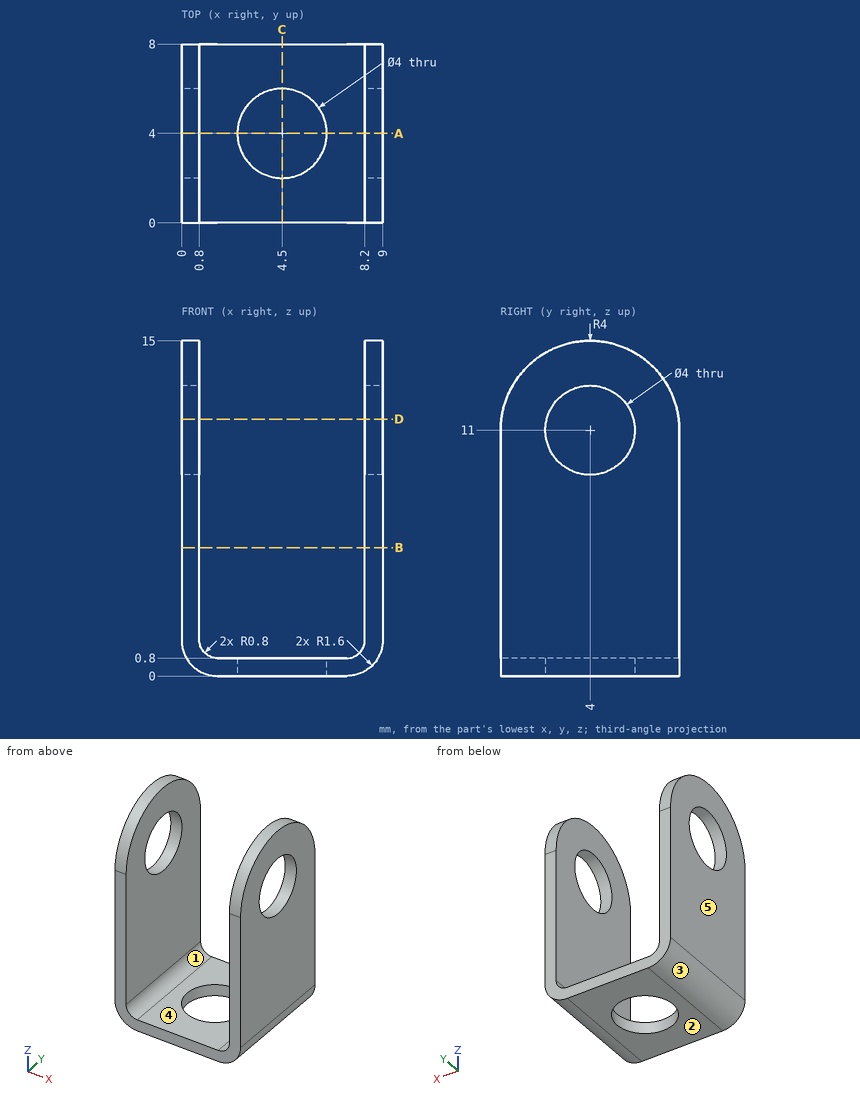
Could you check a few things on this drawing? It's one solid part, dimensions in mm from its lowest x, y, z. A direction names the side the tool comes from. Give positions to 0.01 mm unless a question says otherwise; leave off trailing zeros. Order: outer loops, then holes, each group sorted by start corner. A loop starts at its lowest first (then second) coordinate and runs counter-clockwise, first axis right, second up. Notation, with made-up numbers: (79, 31.5) - (97, 31.5) arc R22 ccw to (97, 42.5) - close; hole circle Ø8 at (-0.75, -35.5). An arc over 180 degrees is marked (long way). One line per question, with ' | ' between items. Start each with the question number.
Item 1: I need wall thicknesses on probe 1 along X at (y, z) = (2.5, 9.5); probe 2 along Y at (x, z) = (0.55, 11); probe 3 along Z at (x, y) = (2.5, 2.25). Which ranges of each line are inside material? Lowest first, please. Write a range as [from, to].
Item 2: I want a section at C-C on x = 4.5. Write out the boundary of the cut face in (y, z), then the cut area to 3 significant figures.
Item 3: Thinking about a two-plate mould opening in X: for the marked faces 1, 2 and 3, which applies, pulls with the +X half, pulls with the -X half, needs draft (parallel to the pull), parting line crosses it, or undercut?
Item 4: I want a section at A-A on y = 4. Write out the boundary of the cut face in (x, z), then the cut area to 3 significant figures.
Item 5: I want a section at B-B on z = 5.75. Write out the boundary of the cut face in (x, y).
Item 6: I want a section at D-D on z = 11.5. Write out the boundary of the cut face in (x, y).
Item 7: I'm going to push flat-ended pins straight in: pin 1 Ø2.5 at (y, z) = (4, 11) entering from -X; pin 2 Ø2 at (x, y) = (6.5, 3.5) entering from +Z; pin 3 Ø1 at (y, z) = (5.5, 7) entering from -X. Where does each tip first touch, or does it pass through?
Item 8: For the marked faces 4 and 5, which set-ups out of +Z, -Z, +X, -X, +Y, -Y let a thin tool reach every point of the face, with its end or its side?
Verdict:
1) probe 1: [0, 0.8], [8.2, 9] | probe 2: [0, 2], [6, 8] | probe 3: [0, 0.8]
2) outline: (0, 0) - (2, 0) - (2, 0.8) - (0, 0.8) - close; (6, 0) - (8, 0) - (8, 0.8) - (6, 0.8) - close | area: 3.20 mm^2
3) face 1: undercut | face 2: needs draft | face 3: pulls with the -X half
4) outline: (0, 1.6) arc R1.6 ccw to (1.6, 0) - (2.5, 0) - (2.5, 0.8) - (1.6, 0.8) arc R0.8 cw to (0.8, 1.6) - (0.8, 9) - (0, 9) - close; (0, 13) - (0.8, 13) - (0.8, 15) - (0, 15) - close; (6.5, 0) - (7.4, 0) arc R1.6 ccw to (9, 1.6) - (9, 9) - (8.2, 9) - (8.2, 1.6) arc R0.8 cw to (7.4, 0.8) - (6.5, 0.8) - close; (8.2, 13) - (9, 13) - (9, 15) - (8.2, 15) - close | area: 19.5 mm^2
5) outline: (0, 0) - (0.8, 0) - (0.8, 8) - (0, 8) - close; (8.2, 0) - (9, 0) - (9, 8) - (8.2, 8) - close
6) outline: (0, 0.03) - (0.8, 0.03) - (0.8, 2.06) - (0, 2.06) - close; (0, 5.94) - (0.8, 5.94) - (0.8, 7.97) - (0, 7.97) - close; (8.2, 0.03) - (9, 0.03) - (9, 2.06) - (8.2, 2.06) - close; (8.2, 5.94) - (9, 5.94) - (9, 7.97) - (8.2, 7.97) - close
7) pin 1: through | pin 2: z = 0.81 | pin 3: x = 0
8) face 4: +Z, +Y, -Y | face 5: +Z, -Z, -X, +Y, -Y
